Source: CAD feature listing. Evaluate the final solid. Frame: model axes, mm. Face numbers are marked on the shaded views. A direction names the side the tool comes from. Coordinates: 2 decimals unless noted, no trailing zeros. Write each loop counter-clockwise with the first axis right and the second up, starting at its lowest first coordinate (ties: lowest second). Pieces come first, ordered by that corner, then holes. Notation, with made-up numbers: (38, 17.5) - (71, 17.5) arc R11 cw to (71, 28.5) - close; hole circle Ø7 at (41.5, 2). An arc over 180 degrees is marked (long way). One line per item, written item: value.
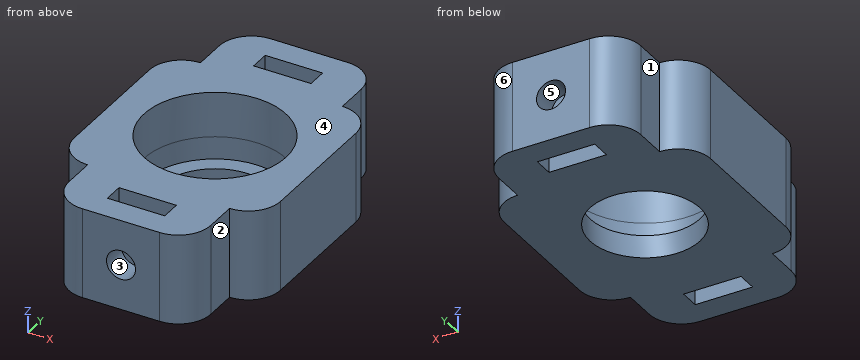
from build123d import *

# Parameters (mm, degrees)
F0_W          = 8.9
F0_H          = 3.1
F0_R          = 11
F1_DEPTH      = 7
F1_DEPTH_BACK = 7
F2_R          = 2.25
F3_DEPTH      = 10
F4_R          = 2.25
F5_DEPTH      = 10
F6_R          = 11.25
F6_R_2        = 8.5
F7_DEPTH      = 3.5


with BuildPart() as f1:
    # F0 (on Top) → F1 (new body, two sides)
    with BuildSketch(Plane.XY) as f1_sk:
        with BuildLine():
            Line((-16, 10), (-16, -10))
            ThreePointArc((-16, -10), (-14.535534, -13.535534), (-11, -15))
            Line((-11, -15), (-11, -20))
            ThreePointArc((-11, -20), (-9.535534, -23.535534), (-6, -25))
            Line((-6, -25), (6, -25))
            ThreePointArc((6, -25), (9.535534, -23.535534), (11, -20))
            Line((11, -20), (11, -15))
            ThreePointArc((11, -15), (14.535534, -13.535534), (16, -10))
            Line((16, -10), (16, 10))
            ThreePointArc((16, 10), (14.535534, 13.535534), (11, 15))
            Line((11, 15), (11, 20))
            ThreePointArc((11, 20), (9.535534, 23.535534), (6, 25))
            Line((6, 25), (-6, 25))
            ThreePointArc((-6, 25), (-9.535534, 23.535534), (-11, 20))
            Line((-11, 20), (-11, 15))
            ThreePointArc((-11, 15), (-14.535534, 13.535534), (-16, 10))
        make_face()
        with Locations((0, -19.45)):
            Rectangle(F0_W, F0_H, mode=Mode.SUBTRACT)
        Circle(F0_R, mode=Mode.SUBTRACT)
        with Locations((0, 19.45)):
            Rectangle(F0_W, F0_H, mode=Mode.SUBTRACT)
    extrude(amount=F1_DEPTH)
    extrude(f1_sk.sketch, amount=-F1_DEPTH_BACK)

    # F2 (on face) → F3 (cut)
    with BuildSketch(Plane.XZ.offset(25)):
        Circle(F2_R)
    extrude(amount=-F3_DEPTH, mode=Mode.SUBTRACT)

    # F4 (on face) → F5 (cut)
    with BuildSketch(Plane(origin=(0, 25, 0), x_dir=(-1, 0, 0), z_dir=(0, 1, 0))):
        Circle(F4_R)
    extrude(amount=-F5_DEPTH, mode=Mode.SUBTRACT)

    # F6 (on face) → F7 (join)
    with BuildSketch(Plane(origin=(0, 0, -7), x_dir=(1, 0, 0), z_dir=(0, 0, -1))):
        Circle(F6_R)
        Circle(F6_R_2, mode=Mode.SUBTRACT)
    extrude(amount=-F7_DEPTH)


solid = f1.part
1) Material intervals for line 1 (Y direction, x = 0, z = 2.5); line 2 (X direction, y = 0, z = -5.5); line 3 (Y direction, x = 4, z = 2), sorted ascending.
Values found:
line 1: -25 to -21, -17.9 to -11, 11 to 17.9, 21 to 25
line 2: -16 to -8.5, 8.5 to 16
line 3: -25 to -21, -17.9 to -10.25, 10.25 to 17.9, 21 to 25
2) Section query D-D on z = 5.5. Output: boundary loops of the cut face in (x, y), then the cut area to 3 significant figures.
Values found:
outline: (-16, -10) arc R5 ccw to (-11, -15) - (-11, -20) arc R5 ccw to (-6, -25) - (6, -25) arc R5 ccw to (11, -20) - (11, -15) arc R5 ccw to (16, -10) - (16, 10) arc R5 ccw to (11, 15) - (11, 20) arc R5 ccw to (6, 25) - (-6, 25) arc R5 ccw to (-11, 20) - (-11, 15) arc R5 ccw to (-16, 10) - close; hole circle Ø22 at (0, 0); hole (-4.45, -21) - (4.45, -21) - (4.45, -17.9) - (-4.45, -17.9) - close; hole (-4.45, 17.9) - (4.45, 17.9) - (4.45, 21) - (-4.45, 21) - close
area: 922 mm2
3) Section query C-C on y = -16.5. Output: boundary loops of the cut face in (x, z).
Values found:
outline: (-11, -7) - (11, -7) - (11, 7) - (-11, 7) - close; hole circle Ø4.5 at (0, 0)
4) Section query A-A on y = 0. Output: boundary loops of the cut face in (x, z).
Values found:
outline: (-16, -7) - (-8.5, -7) - (-8.5, -3.5) - (-11, -3.5) - (-11, 7) - (-16, 7) - close; (8.5, -7) - (16, -7) - (16, 7) - (11, 7) - (11, -3.5) - (8.5, -3.5) - close
5) Section query B-B on x = 7.5. Output: boundary loops of the cut face in (y, z), then the cut area to 3 significant figures.
Values found:
outline: (-24.77, -7) - (-4, -7) - (-4, -3.5) - (-8.05, -3.5) - (-8.05, 7) - (-24.77, 7) - close; (4, -7) - (24.77, -7) - (24.77, 7) - (8.05, 7) - (8.05, -3.5) - (4, -3.5) - close
area: 497 mm2
6) Reachability of the marked faces 1, 2 and 3 from +Z, -Z, +X, -X, +Y, -Y: full face, straight path, thin tool, end or side. Return the list, or none.
Values found:
face 1: +Z, -Z, -X, +Y
face 2: +Z, -Z, +X, -Y
face 3: -Y
7) Contact query for flat-ended pins moving along their axis: P1, Ø3.5, axis at y = -19, z = -2, coming from the -X side; P2, Ø1.5, axis at y = -16.5, z = -1.5, coming from the +X side; P3, Ø10, axis at x = 0, y = 0, coming from the +Z side; P4, Ø17.5, axis at x = 0, y = 0, coming from the +Z side. Output: stop coordinate, or through.
Values found:
P1: x = -11
P2: x = 11
P3: through
P4: z = -3.5
8) Draft query along X for the marked faces 4, 5 and 6. Return one class per face: released by +X, released by -X, zero draft, split by the parting line, or undercut.
Values found:
face 4: zero draft
face 5: undercut
face 6: released by +X
